Could you check a few things on this model? Use its own coordinates, in mm. Give positions to 0.01 mm unless a question says otherwise; leave off trailing zeros. Answer in a Markdown table with one row per item. Add a question column.
```python
from build123d import *

# Parameters (mm, degrees)
SKETCH1_R           = 1
BOSS_EXTRUDE1_DEPTH = 3.7


with BuildPart() as part:
    # Sketch1 → Boss-Extrude1 (new body)
    with BuildSketch(Plane.XY):
        with BuildLine():
            Line((0, -5), (35, -5))
            ThreePointArc((35, -5), (39.915195567, -0.91698012), (36.802854648, 4.663658984))
            add(Edge.make_bspline(
                [(-4.182897753, -2.131172107), (-5.422528099, 19.74118681), (36.802854648, 4.663658984)],
                knots=[0, 0, 0, 1, 1, 1], degree=2))
            ThreePointArc((-4.182897753, -2.131172107), (-2.536080001, -4.213880968), (0, -5))
        make_face()
        with Locations((-2, 0)):
            Circle(SKETCH1_R, mode=Mode.SUBTRACT)
        with Locations((7, 0)):
            Circle(SKETCH1_R, mode=Mode.SUBTRACT)
    extrude(amount=BOSS_EXTRUDE1_DEPTH)


solid = part.part
```
1. Will these pins go through, and if not, where does the flat tip stop? P1, Ø2, axis at y = 1.5, z = 2.5, coming from the -X side; P2, Ø1, axis at y = 3, z = 1.5, coming from the -X side.
2. Suppose I cut it at A-A on y = 0. Count the separate pieces of the cut face and the enclosed holes in it, plus the area to 3 significant figures.
3. If I drill on line 1 along Y through (x, z) = (-2, 2); line 2 along Y through (x, z) = (7, 2.8); line 3 along X through (y, z) = (1.25, 2.35), over which ranges is the centre line in solid material (lowest first)? Write a range as [from, to].
4. Thinking about a two-plate mould opening in X: for faces 1 (the flat face through (17, -5, 2)), 2 (the cylindrical face through (-2.57, -4.19, 1.82)), 3 (the cylindrical face through (6.2, -0.6, 1.8)), 4 (the cylindrical face through (39.9, -1, 1.8)), which applies, pulls with the +X half, pulls with the -X half, needs draft (parallel to the pull), parting line crosses it, or undercut?
Findings below:
| question | item | result |
|---|---|---|
| 1 | P1 | x = -4.16 |
| 1 | P2 | x = -3.87 |
| 2 | separate pieces | 3 |
| 2 | enclosed holes | 0 |
| 2 | area | 149 mm2 |
| 3 | line 1 | [-4.53, -1], [1, 6.61] |
| 3 | line 2 | [-5, -1], [1, 10.7] |
| 3 | line 3 | [-4.09, 39.84] |
| 4 | face 1 | needs draft |
| 4 | face 2 | pulls with the -X half |
| 4 | face 3 | undercut |
| 4 | face 4 | pulls with the +X half |
